Autodesk Inventor part; units mm, degrees
ref_plane "Start Plane" through (0, 0, -6.1539) normal (0, 0, 1) x (1, 0, 0)
ref_plane "End Plane" through (0, 0, 352.6196) normal (0, 0, 1) x (1, 0, 0)
ref_plane "Work Plane4" through (2.3628, -10.403, 355.1877) normal (-0.1481, 0.6522, 0.7434) x (0.9874, 0.0554, 0.1481)
ref_plane "Start Plane" through (0, 0, -6.1539) normal (0, 0, 1) x (1, 0, 0)
ref_plane "End Plane" through (0, 0, 352.6196) normal (0, 0, 1) x (1, 0, 0)
sketch "Sketch" plane through (0, 0, 0) normal (0, 0, 1) x (1, 0, 0)
  circle A0 centre (0, 0) radius 6.9342
  circle A1 centre (0, 0) radius 10.668
  dimension "d0" = 21.336
  dimension "d1" = 3.7338
extrude "Body" add sketch "Sketch" along normal up to surface (358.7736 mm away) from surface at -6.1539
sketch "Sketch3" plane through (0, 0, 0) normal (0, 0, 1) x (1, 0, 0)
  line L0 (0, 0) -> (10, 0)
ref_plane "Work Plane3" through (0, 0, 0) normal (0, -1, 0) x (1, 0, 0)
sketch "Sketch4" plane through (0, 0, 0) normal (0, -1, 0) x (1, 0, 0)
  line L0 (-2, -6.1539) -> (12, -6.1539)
  line L1 (-2, 352.6196) -> (12, 352.6196)
  dimension "d7" = 358.7736
ref_plane "Work Plane4" through (2.3628, -10.403, 355.1877) normal (-0.1481, 0.6522, 0.7434) x (0.9874, 0.0554, 0.1481)
split "Split1" plane through (2.3628, -10.403, 355.1877) removes the side toward (-0.1481, 0.6522, 0.7434)
ref_plane "Work Plane5" through (-10.4409, -2.1896, 359.7619) normal (0.7819, 0.164, 0.6014) x (0.6182, -0.0801, -0.7819)
split "Split2" plane through (-10.4409, -2.1896, 359.7619) removes the side toward (0.7819, 0.164, 0.6014)
ref_plane "Work Plane6" through (-9.9997, 3.7164, 387.2134) normal (0.908, -0.3375, 0.2483) x (0.3395, 0.2455, -0.908)
split "Split3" plane through (-9.9997, 3.7164, 387.2134) removes the side toward (0.908, -0.3375, 0.2483)
ref_plane "Work Plane7" through (2.3628, -10.403, -11.8569) normal (-0.1647, 0.7249, -0.6689) x (0.9181, 0.3604, 0.1647)
split "Split4" plane through (2.3628, -10.403, -11.8569) removes the side toward (-0.1647, 0.7249, -0.6689)
ref_plane "Work Plane8" through (-9.9997, 3.7164, -14.2686) normal (0.7507, -0.279, -0.5988) x (-0.4048, 0.5221, -0.7507)
split "Split5" plane through (-9.9997, 3.7164, -14.2686) removes the side toward (0.7507, -0.279, -0.5988)
ref_plane "Work Plane9" through (-9.9328, -3.8919, -6.776) normal (0.4992, 0.1956, -0.8441) x (-0.5987, -0.6264, -0.4992)
split "Split6" plane through (-9.9328, -3.8919, -6.776) removes the side toward (0.4992, 0.1956, -0.8441)
equation "\"d0\" = G_H"
equation "\"d1\" = G_T"
equation "\"d2\" = G_L"
equation "\"G_H\" = 21.336"
equation "\"G_T\" = 3.7338"
equation "\"G_L\" = 358.77357"
equation "\"G_OFFSET_START\" = 6.15394"
equation "\"G_OFFSET_END\" = 7.03027"
equation "\"d4\" = -G_OFFSET_START"
equation "\"d5\" = G_OFFSET_END + B_L"
equation "\"B_L\" = 345.58937"
properties part number "ANSI - 1/2 x 0.147 - 14.125" material "Steel, Mild"
Input: part model. Units: mm. Frame: model coordinates. Give positions to 0.01 mm unless a question says otherwise; leave off trailing zeros. Order: outer loops, then holes, each group sorted by start corner. A loop starts at its lowest first (then second) coordinate and runs counter-clockwise, first axis right, second up. Notation, with made-up numbers: M -38.5,18 L -33.5,18 A19 cw -33.5,39 Z; hole C 0.5,83 d7. An arc over 180 degrees is marked long. One line per question, with ' | ' between items.
1) Draft query along Y for faces 1 (the face through (-5.5, 4.22, 170.6)), 2 (the face through (-5.634, 4.674, 6.451)), 3 (the face through (4.175, -6.071, 8.061)). Return one class per face: pulls with the +Y half, pulls with the -Y half, needs draft (parallel to the pull), parting line crosses it, or undercut.
Filled in:
face 1: undercut | face 2: pulls with the +Y half | face 3: pulls with the -Y half
2) Section B-B on z = 69. Output: boundary loops of the cut face in (x, y), and give its area (3 significant figures).
Filled in:
outline: C 0,0 d21.34; hole C 0,0 d13.87 | area: 206 mm2
3) Ray query, L1, parallel to X at y = 0, z = 262; L2, parallel to Y at x = -4, z = 337.5. Return the intervals inside material, ascending.
Filled in:
L1: x = -10.67 to -6.93, 6.93 to 10.67 | L2: y = -9.89 to -5.66, 5.66 to 8.31
4) Contact query for flat-ended pins moving along their axis: P1, Ø10, axis at y = 6.5, z = 231.5, coming from the -X side; P2, Ø2, axis at x = 3, z = 161.5, coming from the -Y side; P3, Ø1.5, axis at x = 3.5, z = 258.5, coming from the +Y side. Output: stop coordinate, or through.
Filled in:
P1: stops at x = -10.56 | P2: stops at y = -10.48 | P3: stops at y = 10.31
5) Section A-A on y = 0. Output: boundary loops of the cut face in (x, z), and give its area (3 significant figures).
Filled in:
outline: M -10.67,2.63 L -6.93,1.71 L -6.93,344.21 L -10.67,343.46 Z; M 6.93,8.69 L 10.67,13.37 L 10.67,306.58 L 6.93,320.24 Z | area: 2,400 mm2
